```python
from build123d import *

# Parameters (mm, degrees)
SKETCH_1_R               = 3.6
EXTRUDE_1_DEPTH          = 10
SKETCH_2_R               = 2
SKETCH_2_R_2             = 1
EXTRUDE_2_DEPTH          = 2
SKETCH_4_R               = 2
EXTRUDE_3_DEPTH          = 2
SKETCH_5_R               = 1.8
EXTRUDE_4_DEPTH          = 3.6
SKETCH_2_3_R             = 1
CUT_EXTRUDE_2_DEPTH      = 3
CUT_EXTRUDE_2_DEPTH_BACK = 13
EXTRUDE_5_DEPTH          = 10
SKETCH_10_W              = 2
SKETCH_10_H              = 2


with BuildPart() as part:
    # Sketch 1 → Extrude 1 (new body)
    with BuildSketch(Plane.XY):
        Circle(SKETCH_1_R)
    extrude(amount=EXTRUDE_1_DEPTH)

    # Sketch 2 → Extrude 2 (add)
    with BuildSketch(Plane.XY.offset(10)):
        Circle(SKETCH_2_R)
        Circle(SKETCH_2_R_2, mode=Mode.SUBTRACT)
    extrude(amount=EXTRUDE_2_DEPTH)

    # Sketch 4 → Extrude 3 (add)
    with BuildSketch(Plane(origin=(0, 0, 0), x_dir=(-1, 0, 0), z_dir=(0, 0, -1))):
        with Locations(Location((0, 0, 0), (0, 0, 180))):  # turned: the seam where the file's is
            Circle(SKETCH_4_R)
    extrude(amount=EXTRUDE_3_DEPTH)

    # Sketch 5 → Extrude 4 (add)
    with BuildSketch(Plane(origin=(0, 0, 0), x_dir=(1, 0, 0), z_dir=(0, 1, 0))):
        with Locations((-1.8, -5)):
            Circle(SKETCH_5_R)
    extrude(amount=EXTRUDE_4_DEPTH)

    # Sketch 2_3 → Cut-Extrude 2 (cut, two sides)
    with BuildSketch(Plane.XY.offset(10)) as cut_extrude_2_sk:
        Circle(SKETCH_2_3_R)
    extrude(amount=CUT_EXTRUDE_2_DEPTH, mode=Mode.SUBTRACT)
    extrude(cut_extrude_2_sk.sketch, amount=-CUT_EXTRUDE_2_DEPTH_BACK, mode=Mode.SUBTRACT)

    # Sketch 8 → Extrude 5 (add)
    with BuildSketch(Plane.XY.offset(10)):
        Polygon((0, 3.6), (-3.6, 0), (-3.6, 3.6), align=None)
    extrude(amount=-EXTRUDE_5_DEPTH)

    # Sweep 1: sweep along a path in Sketch 11
    with BuildLine(Plane.XY.offset(5)) as sweep_1_path:
        Line((-2.6, 3.6), (-2.6, 1.5011107))
        Line((-2.6, 1.5011107), (0, 0))
    # Sketch 10 → Sweep 1 (sweep, cut)
    with BuildSketch(Plane(origin=(0, 3.6, 0), x_dir=(1, 0, 0), z_dir=(0, 1, 0))):
        with Locations((-2.6, -5)):
            Rectangle(SKETCH_10_W, SKETCH_10_H)
    sweep(path=sweep_1_path.line, transition=Transition.RIGHT, mode=Mode.SUBTRACT)


solid = part.part
```
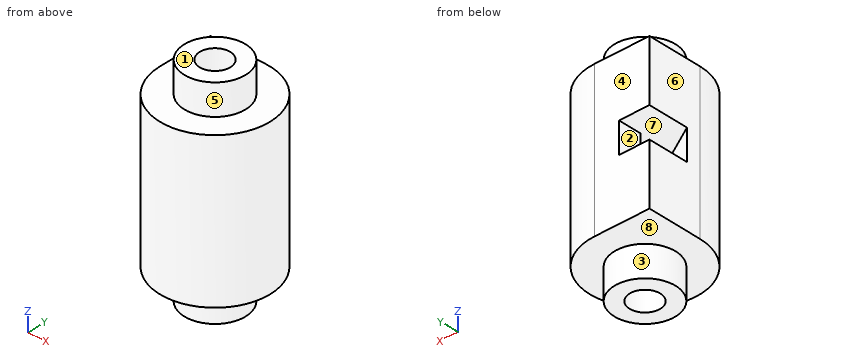
Check sheet for the modelled part. Datum: model origin and axes. Units: mm. Face numbers are marked on the shaded views. A direction names the side the tool comes from. Coordinates: 2 decimals unless noted, no trailing zeros. Order: outer loops, then holes, each group sorted by start corner. A loop starts at its lowest first (then second) coordinate and runs counter-clockwise, first axis right, second up. Notation, with made-up numbers: (-29.5, 77.25) -> (12.5, 77.25) arc R21 cw to (12.5, 93.25) -> close; hole circle Ø5 at (52.25, -17.75). An arc over 180 degrees is marked (long way). Write each question's results on one line, items separated by ' | '. Start each with the question number.
1) Section check B-B (y = 0.5). Enter the section's corners in (x, z).
2) Section check A-A (z = 4.25). Enter the section's corners in (x, y).
3) Draft check along Z on the marked faces 6, 7 and 8. Enter one of: pulls with the +Z half, pulls with the -Z half, needs draft (parallel to the pull), parting line crosses it, or undercut.
4) Depth check by flat-ended pin: pin 1 (2 mm diameter, centred on x = 2.5, z = 2.5, fed in from +Y); pin 2 (3 mm diameter, centred on y = -2.5, z = 2, fed in from +X); pin 3 (1.2 mm diameter, centred on y = 3, z = 5, fed in from -X); pin 4 (2 mm diameter, centred on x = 1, z = 3.5, fed in from +Y). Enter the tip coordinate at first touch or a pass-through.
5) Set-up check for the marked faces 1, 2, 3, 4 and 5: record each of +Z, -Z, +X, -X, +Y, -Y from which the full face is reachable in a straight line by a thin tool's end or side.
6) Section check D-D (z = 8). Enter the section's corners in (x, y).
7) Section check C-C (y = 1.75). Enter the section's corners in (x, z).
8) Material ranges on line 1 along X through (y, z) = (0, 5); line 2 along Y through (x, z) = (0, 1.5); line 3 along Y through (x, z) = (0, 10.8), recorded low to high.
Checked values:
1) outline: (-3.6, 0) -> (-1.94, 0) -> (-1.94, -2) -> (-0.87, -2) -> (-0.87, 4) -> (-2.87, 4) -> (-2.87, 6) -> (-0.87, 6) -> (-0.87, 12) -> (-1.94, 12) -> (-1.94, 10) -> (-3.6, 10) -> close; (0.87, -2) -> (1.94, -2) -> (1.94, 0) -> (3.57, 0) -> (3.57, 10) -> (1.94, 10) -> (1.94, 12) -> (0.87, 12) -> close
2) outline: (-3.6, 0) arc R3.6 ccw (long way) to (0, 3.6) -> (-1.6, 3.6) -> (-1.6, 2.08) -> (0.5, 0.87) arc R1 cw to (-0.5, -0.87) -> (-3.6, 0.92) -> close
3) face 6: needs draft | face 7: undercut | face 8: pulls with the -Z half
4) pin 1: y = 3.27 | pin 2: x = 3.46 | pin 3: x = -1.6 | pin 4: y = 3.6
5) face 1: +Z, +X, -X, +Y, -Y | face 2: -X, +Y | face 3: -Z | face 4: +Z, -Z, +X, -X, +Y | face 5: +Z
6) outline: (-3.6, 0) arc R3.6 ccw (long way) to (0, 3.6) -> (-3.6, 3.6) -> close; hole circle Ø2 at (0, 0)
7) outline: (-3.6, 0) -> (-0.97, 0) -> (-0.97, -2) -> (0.97, -2) -> (0.97, 0) -> (3.15, 0) -> (3.15, 10) -> (0.97, 10) -> (0.97, 12) -> (-0.97, 12) -> (-0.97, 10) -> (-3.6, 10) -> (-3.6, 6) -> (-1.03, 6) -> (-1.03, 4) -> (-3.6, 4) -> close
8) line 1: -3.6 to -2, 1 to 3.6 | line 2: -3.6 to -1, 1 to 3.6 | line 3: -2 to -1, 1 to 2
